The listing builds one solid part. Answer for the finished solid, in the listing's coordinates (mm). Face numbers are marked on the shaded views. A direction names the side the tool comes from. Give positions to 0.01 mm unless a question says otherwise; leave off trailing zeros. Order: outer loops, then holes, each group sorted by start corner. A loop starts at its lowest first (then second) coordinate and runs counter-clockwise, first axis right, second up.
```python
from build123d import *

# Parameters (mm, degrees)
F0_W     = 254
F0_H     = 152.4
F1_DEPTH = 38.1
F2_W     = 228.6844402552
F2_H     = 123.7743124366
F3_DEPTH = 63.5


with BuildPart() as f1:
    # F0 (on Top) → F1 (new body, symmetric)
    with BuildSketch(Plane.XY):
        Rectangle(F0_W, F0_H)
    extrude(amount=F1_DEPTH, both=True)

    # F2 (on face) → F3 (cut)
    with BuildSketch(Plane.XY.offset(38.1)):
        Rectangle(F2_W, F2_H)
    extrude(amount=-F3_DEPTH, mode=Mode.SUBTRACT)


solid = f1.part
```
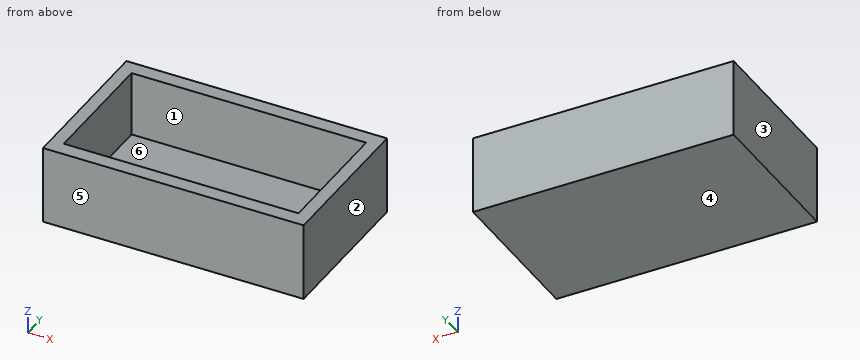
1) Find section C-C (x = -15.5). Write down the section's boundary in (y, z), then the cut area to 3 significant figures.
Geometry says:
outline: (-76.2, -38.1) - (76.2, -38.1) - (76.2, 38.1) - (61.89, 38.1) - (61.89, -25.4) - (-61.89, -25.4) - (-61.89, 38.1) - (-76.2, 38.1) - close
area: 3,750 mm2
2) For a pull along X with two mould halves and no side action, classify the marked faces 1, 2, 3 and 4 as +X half, -X half, draft (parallel to the pull), parting line (faces both ways), or undercut.
Geometry says:
face 1: undercut
face 2: +X half
face 3: -X half
face 4: draft
3) Find section B-B (z = -4). Write down the section's boundary in (x, y).
Geometry says:
outline: (-127, -76.2) - (127, -76.2) - (127, 76.2) - (-127, 76.2) - close; hole (-114.34, -61.89) - (114.34, -61.89) - (114.34, 61.89) - (-114.34, 61.89) - close
4) Straight lines are drawn through the part: probe 1 along Y at (x, z) = (-97, 29.5); probe 2 along X at (y, z) = (50.5, -23.5); probe 3 along Z at (x, y) = (-57, 57). For each, find the intervals that lie inside material, in ascending order.
Geometry says:
probe 1: y = -76.2 to -61.89, 61.89 to 76.2
probe 2: x = -127 to -114.34, 114.34 to 127
probe 3: z = -38.1 to -25.4
5) Find section A-A (y = 1.5). Write down the section's boundary in (x, z), then the cut area to 3 significant figures.
Geometry says:
outline: (-127, -38.1) - (127, -38.1) - (127, 38.1) - (114.34, 38.1) - (114.34, -25.4) - (-114.34, -25.4) - (-114.34, 38.1) - (-127, 38.1) - close
area: 4,830 mm2
6) Given P1, Ø5, axis at x = 54.5, y = -17, coming from the +Z side, flat-ended and moving along its own axis, determine where the tip first touches the part or whether it passes through.
Geometry says:
P1: stops at z = -25.4
7) A tool of negligible diameter and unlimited length cuts with its end or side. For the marked faces 5 and 6, from which of +Z, -Z, +X, -X, +Y, -Y can it reach the whole face along a straight path? Write none if from no direction.
Geometry says:
face 5: +Z, -Z, +X, -X, -Y
face 6: +Z
